Drawing for the job (mm, zero at the part's lowest x, y, z). Coordinates: 2 decimals unless noted, no trailing zeros. Loops run counter-clockwise (first coordinate to the right, second up) from the corner with the lowest first, then second, coordinate; pieces in that order, holes last. Notation, with made-up numbers: (65.25, 71) - (114.25, 71) arc R25 cw to (114.25, 89) - close; hole circle Ø11 at (24, -1). An arc over 180 degrees is marked (long way). One line per item, written item: value.
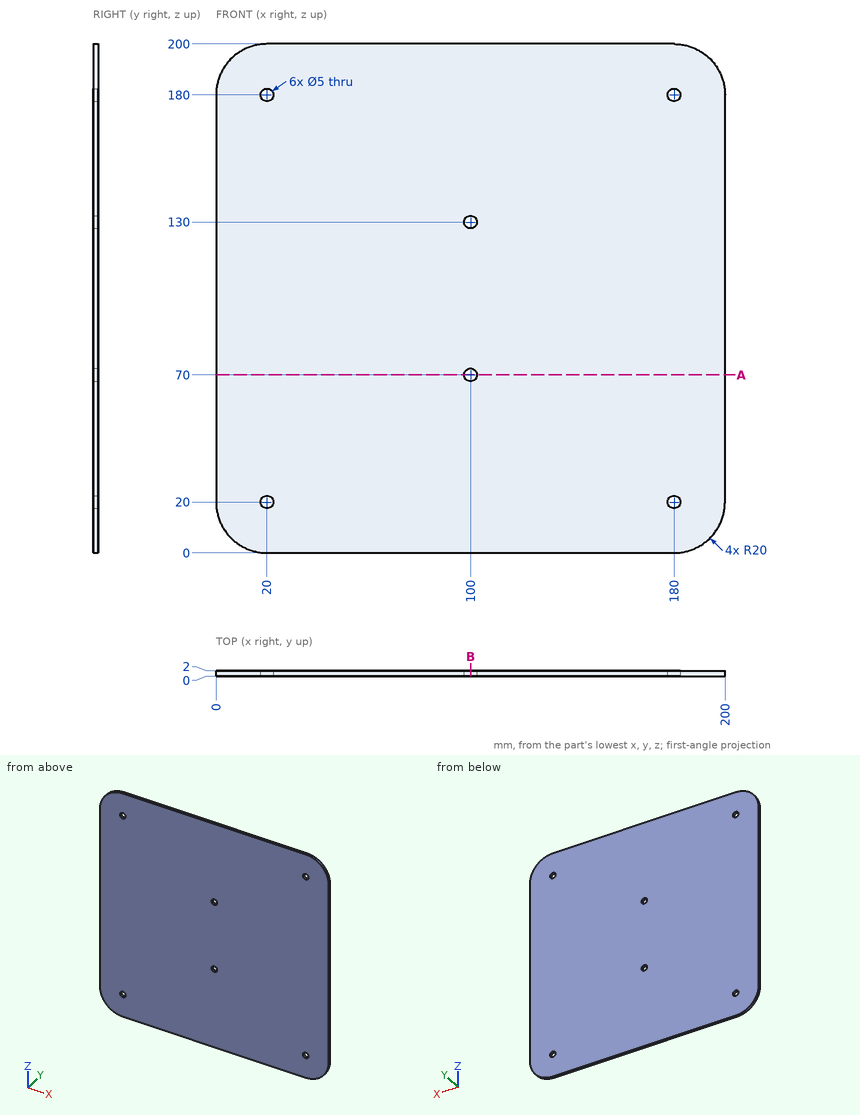
Item 1: Drop a flat-ended pin along its axis: P1, Ø4, axis at x = 100, z = 70, coming from the -Y side. Give the stop position or say it passes through.
Check result:
P1: passes through
Item 2: Cut at B-B, the plane x = 100. Write the cut outline in (y, z).
Check result:
outline: (0, 0) - (2, 0) - (2, 67.5) - (0, 67.5) - close; (0, 72.5) - (2, 72.5) - (2, 127.5) - (0, 127.5) - close; (0, 132.5) - (2, 132.5) - (2, 200) - (0, 200) - close
Item 3: Probe probe 1 along X at (y, z) = (1.15, 20); probe 2 along Z at (x, y) = (100, 0.6). List the from-to ranges inside material, lowest first. Write a range as from..to.
Check result:
probe 1: x = 0..17.5, 22.5..177.5, 182.5..200
probe 2: z = 0..67.5, 72.5..127.5, 132.5..200
Item 4: Cut at A-A, the plane z = 70. Write the cut outline in (x, y), then the cut area to 3 significant figures.
Check result:
outline: (0, 0) - (97.5, 0) - (97.5, 2) - (0, 2) - close; (102.5, 0) - (200, 0) - (200, 2) - (102.5, 2) - close
area: 390 mm^2
